from build123d import *

# Parameters (mm, degrees)
F1_DEPTH = 914.4
F3_D     = 25.4
F3_DEPTH = 101.6
F3_TIP   = 7.6309298617
F4_D     = 25.4
F4_DEPTH = 304.8
F4_TIP   = 7.6309298617


with BuildPart() as f1:
    # F0 (on Right) → F1 (new body)
    with BuildSketch(Plane.YZ):
        with BuildLine():
            Line((6.3090295458, 1012.4358065891), (1.2290295458, 1012.4358065891))
            ThreePointArc((1.2290295458, 1012.4358065891), (-32.8959437143, 998.3007798492), (-47.0309704542, 964.1758065891))
            Line((-47.0309704542, 964.1758065891), (-47.0309704542, 44.6958065891))
            ThreePointArc((-47.0309704542, 44.6958065891), (-32.8959437143, 10.5708333291), (1.2290295458, -3.5641934109))
            Line((1.2290295458, -3.5641934109), (6.3090295458, -3.5641934109))
            ThreePointArc((6.3090295458, -3.5641934109), (40.4340028058, 10.5708333291), (54.5690295458, 44.6958065891))
            Line((54.5690295458, 44.6958065891), (54.5690295458, 964.1758065891))
            ThreePointArc((54.5690295458, 964.1758065891), (40.4340028058, 998.3007798492), (6.3090295458, 1012.4358065891))
        make_face()
    extrude(amount=F1_DEPTH)

    # F3
    with Locations(Plane.XY.offset(1012.4358065891)):
        with Locations((50.8, 3.7690295458)):
            Hole(F3_D / 2, depth=F3_DEPTH)
            with Locations((0, 0, -(F3_DEPTH + F3_TIP / 2))):  # 118° drill point
                Cone(0, F3_D / 2, F3_TIP, mode=Mode.SUBTRACT)

    # F4
    with Locations(Plane.XY.offset(1012.4358065891)):
        with Locations((863.6, 3.7690295458)):
            Hole(F4_D / 2, depth=F4_DEPTH)
            with Locations((0, 0, -(F4_DEPTH + F4_TIP / 2))):  # 118° drill point
                Cone(0, F4_D / 2, F4_TIP, mode=Mode.SUBTRACT)


solid = f1.part
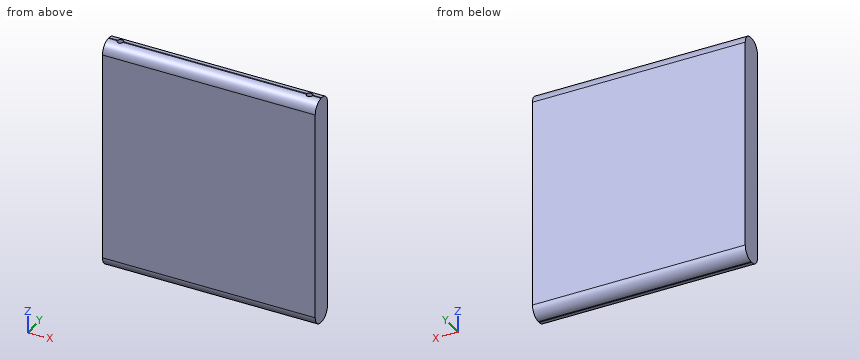
Geometry: final body of the model. Coordinates: model frame, mm. Give positions to 0.01 mm unless a question says otherwise; leave off trailing zeros. Write each loop counter-clockwise with the first axis right and the second up, starting at its lowest first coordinate (ties: lowest second). Pieces come first, ordered by that corner, then holes. Notation, with made-up numbers: (-1, -2.75) - (9, -2.75) arc R24 ccw to (9, 15.25) - close; hole circle Ø11 at (-17.75, -13.75). An arc over 180 degrees is marked (long way). Return JSON: item names as keys, results as strings. Group by question number.
1) Section A-A on x = 676. Return the cut outline in (y, z), plus the area to 3 significant figures.
2) Line query: line 1 (Y direction, x = 863, z = 811); line 2 (Y direction, x = 50, z = 974); line 3 (Z direction, x = 563, y = -18). Output: solid intervals per line, ascending.
3) First-contact query: P1, Ø1, axis at x = 361, y = -12, coming from the +Z side; P2, Ø3, axis at x = 220.5, y = 43, coming from the +Z side; P3, Ø15, axis at x = 863.6, y = 3.77, coming from the +Z side. Flat tips, straight axial feed; report the tip coordinate or a pass-through.
Filled in:
{
 "1": {"outline": "(-47.03, 44.7) arc R48.26 ccw to (1.23, -3.56) - (6.31, -3.56) arc R48.26 ccw to (54.57, 44.7) - (54.57, 964.18) arc R48.26 ccw to (6.31, 1012.44) - (1.23, 1012.44) arc R48.26 ccw to (-47.03, 964.18) - close", "area": "101,000 mm^2"},
 "2": {"line 1": "y = -47.03 to -8.92, 16.45 to 54.57", "line 2": "y = -46.02 to -8.91, 16.44 to 53.56", "line 3": "z = 0.43 to 1008.44"},
 "3": {"P1": "stops at z = 1010.73", "P2": "stops at z = 997.2", "P3": "stops at z = 704.51"}
}
